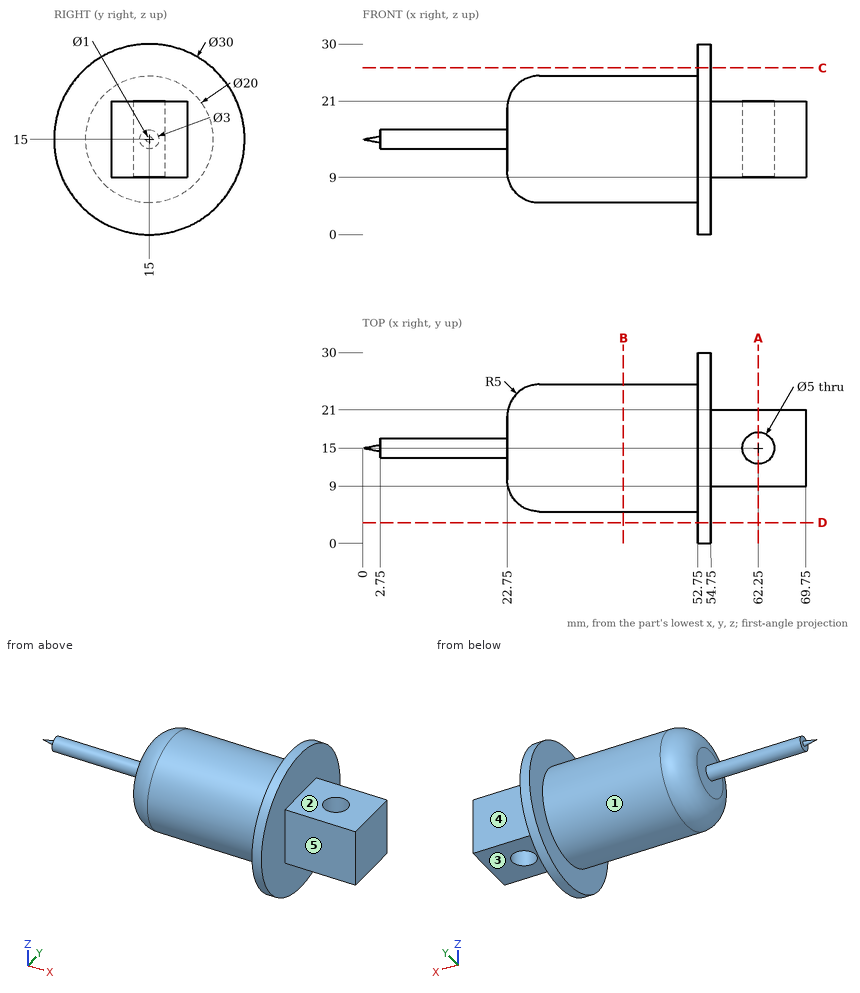
The figure shows three views and two pictorial views of one solid part (mm, origin at its lowest corner). Answer the questions. A direction names the side the tool comes from. Give positions to 0.01 mm unless a question says otherwise; leave off trailing zeros. Order: outer loops, then holes, each group sorted by start corner. A loop starts at its lowest first (then second) coordinate and runs counter-clockwise, first axis right, second up. Notation, with made-up numbers: (13.5, 62) - (53.5, 62) arc R19 ccw to (53.5, 66) - close; hole circle Ø2 at (68.5, 80). An arc over 180 degrees is marked (long way). Answer as CSV lines item,"result".
Q1. A cutting plane is placed at D-D, the plane y = 3.25. Determine the outline of the cut face in (x, z).
Answer key:
outline,"(52.75, 5.68) - (54.75, 5.68) - (54.75, 24.32) - (52.75, 24.32) - close"
Q2. A cutting plane is placed at A-A, the plane x = 62.25. Determine the outline of the cut face in (y, z), and give its area (3 significant figures).
Answer key:
outline,"(9, 9) - (12.5, 9) - (12.5, 21) - (9, 21) - close; (17.5, 9) - (21, 9) - (21, 21) - (17.5, 21) - close"
area,"84.0 mm^2"
Q3. A cutting plane is placed at B-B, the plane x = 41. Determine the outline of the cut face in (y, z).
Answer key:
outline,"circle Ø20 at (15, 15)"
Q4. A cutting plane is placed at C-C, the plane z = 26.25. Determine the outline of the cut face in (x, y), and give its area (3 significant figures).
Answer key:
outline,"(52.75, 5.08) - (54.75, 5.08) - (54.75, 24.92) - (52.75, 24.92) - close"
area,"39.7 mm^2"
Q5. Straight lines are drawn through the part: L1, parallel to X at y = 15, z = 12.5; L2, parallel to X at y = 15, z = 15.75; L3, parallel to X at y = 19, z = 3.5. For each, find the intervals that lie inside material, in ascending order.
Answer key:
L1,"x = 22.75 to 59.75, 64.75 to 69.75"
L2,"x = 2.75 to 59.75, 64.75 to 69.75"
L3,"x = 52.75 to 54.75"
Q6. Each of these flat-tipped pins is pushed along its axis until it touches: pin 1 Ø6 at (x, y) = (62.25, 15) entering from +Z; pin 2 Ø3.5 at (x, z) = (60, 17.5) entering from -Y; pin 3 Ø6 at (x, y) = (58.5, 12.5) entering from -Z. Where does it stop, or does it pass through?
Answer key:
pin 1,"stops at z = 21"
pin 2,"stops at y = 9"
pin 3,"stops at z = 9"
Q7. Which of the six approach directions +Z, -Z, +X, -X, +Y, -Y give full straight-line access (tool end or side, diameter ignored) to the marked faces 1, 2, 3, 4 and 5?
Answer key:
face 1,"-X"
face 2,"+Z, +X, +Y, -Y"
face 3,"-Z, +X, +Y, -Y"
face 4,"+Z, -Z, +X, +Y"
face 5,"+Z, -Z, +X, -Y"
